```python
from build123d import *

# Parameters (mm, degrees)
BOSS_EXTRUDE1_DEPTH = 30
BOSS_EXTRUDE2_DEPTH = 3
FILLET1_R           = 4
SKETCH4_R           = 0.75
CUT_EXTRUDE1_DEPTH  = 3
SKETCH9_R           = 0.75
CUT_EXTRUDE4_DEPTH  = 3
SKETCH6_R           = 0.75
CUT_EXTRUDE3_DEPTH  = 3
BOSS_EXTRUDE3_DEPTH = 5
SKETCH10_W          = 2.3
SKETCH10_H          = 2.3
CUT_EXTRUDE5_DEPTH  = 3


with BuildPart() as part:
    # Sketch1 → Boss-Extrude1 (new body)
    with BuildSketch(Plane(origin=(0, 0, 0), x_dir=(1, 0, 0), z_dir=(0, 1, 0))):
        Polygon((14.623899198, -62.06566226), (4.913523379, -35.386623963), (96.462113254, -2.06566226), (74.623899198, -62.06566226), align=None)
        Polygon((16.724521813, -59.06566226), (8.758661672, -37.179641396), (91.442641699, -7.085133815), (72.523276583, -59.06566226), align=None, mode=Mode.SUBTRACT)
    extrude(amount=BOSS_EXTRUDE1_DEPTH)

    # Sketch3 → Boss-Extrude2 (add)
    with BuildSketch(Plane(origin=(0, 0, 0), x_dir=(1, 0, 0), z_dir=(0, 1, 0))):
        Polygon((8.758661672, -37.179641396), (16.724521813, -59.06566226), (72.523276583, -59.06566226), (91.442641699, -7.085133815), align=None)
    extrude(amount=BOSS_EXTRUDE2_DEPTH)

    # Fillet1
    fillet1_edges = [part.edges().sort_by_distance(p)[0] for p in [
        (91.442641699, 16.5, 7.085133815),
        (8.758661672, 16.5, 37.179641396),
        (9.768711289, 0, 48.726143111),
        (50.687818317, 0, 18.726143111),
        (85.543006226, 0, 32.06566226),
        (4.913523379, 15, 35.386623963),
        (96.462113254, 15, 2.06566226),
    ]]
    fillet(fillet1_edges, radius=FILLET1_R)

    # Sketch4 → Cut-Extrude1 (cut)
    with BuildSketch(Plane(origin=(11.947814765, 0, 32.826351279), x_dir=(-0.939692621, 0, 0.342020143), z_dir=(-0.342020143, 0, -0.939692621))):
        with Locations((-71.514263462, 15.5)):
            Circle(SKETCH4_R)
        with Locations((-51.514263462, 15.5)):
            Circle(SKETCH4_R)
        with Locations((-31.514263462, 15.5)):
            Circle(SKETCH4_R)
        with Locations((-11.514263462, 15.5)):
            Circle(SKETCH4_R)
        with Locations((-11.514263462, 6)):
            Circle(SKETCH4_R)
        with Locations((-31.514263462, 6)):
            Circle(SKETCH4_R)
        with Locations((-51.514263462, 6)):
            Circle(SKETCH4_R)
        with Locations((-71.514263462, 6)):
            Circle(SKETCH4_R)
    extrude(amount=-CUT_EXTRUDE1_DEPTH, mode=Mode.SUBTRACT)

    # Sketch9 → Cut-Extrude4 (cut)
    with BuildSketch(Plane(origin=(85.842080595, 0, 31.243962184), x_dir=(0.342020143, 0, -0.939692621), z_dir=(0.939692621, 0, 0.342020143))):
        with Locations((-17.79976813, 15.5)):
            Circle(SKETCH9_R)
        with Locations((-17.79976813, 6)):
            Circle(SKETCH9_R)
    extrude(amount=-CUT_EXTRUDE4_DEPTH, mode=Mode.SUBTRACT)

    # Sketch6 → Cut-Extrude3 (cut)
    with BuildSketch(Plane.XY.offset(62.06566226)):
        with Locations((34.623899198, 25)):
            Circle(SKETCH6_R)
        with Locations((44.623899198, 25)):
            Circle(SKETCH6_R)
        with Locations((54.623899198, 25)):
            Circle(SKETCH6_R)
        with Locations((64.623899198, 25)):
            Circle(SKETCH6_R)
        with Locations((34.623899198, 15.5)):
            Circle(SKETCH6_R)
        with Locations((44.623899198, 15.5)):
            Circle(SKETCH6_R)
        with Locations((54.623899198, 15.5)):
            Circle(SKETCH6_R)
        with Locations((64.623899198, 15.5)):
            Circle(SKETCH6_R)
        with Locations((24.623899198, 25)):
            Circle(SKETCH6_R)
        with Locations((24.623899198, 15.5)):
            Circle(SKETCH6_R)
    extrude(amount=-CUT_EXTRUDE3_DEPTH, mode=Mode.SUBTRACT)

    # Sketch7 → Boss-Extrude3 (add)
    with BuildSketch(Plane.XY.offset(62.06566226)):
        with BuildLine():
            Line((37.623899198, 9), (51.623899198, 9))
            ThreePointArc((51.623899198, 9), (54.623899198, 6), (51.623899198, 3))
            Line((51.623899198, 3), (37.623899198, 3))
            ThreePointArc((37.623899198, 3), (34.623899198, 6), (37.623899198, 9))
        make_face()
    extrude(amount=BOSS_EXTRUDE3_DEPTH)

    # Sketch10 → Cut-Extrude5 (cut)
    with BuildSketch(Plane(origin=(85.842080595, 0, 31.243962184), x_dir=(0.342020143, 0, -0.939692621), z_dir=(0.939692621, 0, 0.342020143))):
        with Locations((-13.79976813, 15.5)):
            Rectangle(SKETCH10_W, SKETCH10_H)
        with Locations((-13.79976813, 6)):
            Rectangle(SKETCH10_W, SKETCH10_H)
    extrude(amount=-CUT_EXTRUDE5_DEPTH, mode=Mode.SUBTRACT)


solid = part.part
```
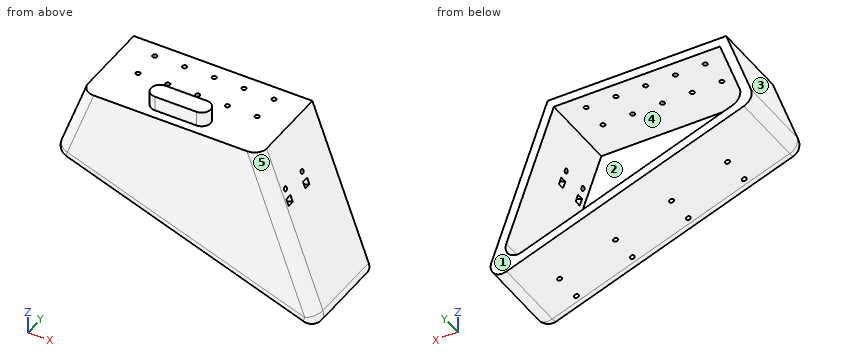
Work out the finished part from the listing and answer in its coordinate system (mm). Face numbers are marked on the shaded views. A direction names the side the tool comes from. Round coordinates to 2 decimals unless told otherwise and drop trailing zeros. Write each loop counter-clockwise with the first axis right and the second up, starting at its lowest first coordinate (ties: lowest second). Pieces come first, ordered by that corner, then holes.
1) Which of the six approach directions +Z, -Z, +X, -X, +Y, -Y give full straight-line access (tool end or side, diameter ignored) to the marked faces 1 and 2?
2) A cutting plane is placed at A-A on y = 19.5. Determine the outline of the cut face in (x, z), and give its area (3 significant figures).
3) Determine the mould class of the marked faces 3, 4 and 5 for opening direction X: pulls with the +X half, pulls with the -X half, needs draft (parallel to the pull), parting line crosses it, or undercut.
4) Flat-ended cylindrical pins translate along their axes: P1, Ø1, axis at y = 9.5, z = 41.5, coming from the +X side; P2, Ø1.6, axis at x = 80.5, z = 44.5, coming from the -Y side; P3, Ø0.9, axis at x = 34.62, y = 25, coming from the -Z side. Find the tip coordinate at first contact, or state that the pin passes through.
5) A cutting plane is placed at B-B on z = 63. Determine the outline of the cut face in (x, y), and give its area (3 significant figures).
6) Consider probe 1 along Y at (x, z) = (41.5, 23); probe 2 along Y at (x, z) = (81, 12.5); probe 3 along Z at (x, y) = (47.5, 23.25). Determine where each line is inside the solid, lowest interval first.
7) A cutting plane is placed at C-C on z = 31. Give the number of separate pieces and of enclosed holes in the cut face, and give its area (3 significant figures).
Entries:
1. face 1: +Z, -Z, +X, -X, +Y
1. face 2: +Y
2. outline: (6.28, 39.15) arc R4 ccw to (8.67, 34.02) - (88.4, 5) arc R4 ccw to (93.53, 10.13) - (74.62, 62.07) - (14.62, 62.07) - close; hole (10.13, 40.94) arc R4 ccw to (12.52, 35.81) - (83.38, 10.02) arc R4 ccw to (88.51, 15.15) - (72.52, 59.07) - (16.72, 59.07) - close
2. area: 708 mm2
3. face 3: pulls with the -X half
3. face 4: undercut
3. face 5: pulls with the +X half
4. P1: stops at x = 82.29
4. P2: stops at y = 1.06
4. P3: stops at z = 24.41
5. outline: (37.62, 3) - (51.62, 3) arc R3 ccw to (51.62, 9) - (37.62, 9) arc R3 ccw to start
5. area: 112 mm2
6. probe 1: y = 1.5 to 5.36, 6.64 to 14.86, 16.14 to 30
6. probe 2: y = 0 to 3
6. probe 3: z = 19.89 to 23.08, 59.07 to 62.07
7. separate pieces: 1
7. enclosed holes: 2
7. area: 512 mm2
